```python
from build123d import *

# Parameters (mm, degrees)
SKETCH1_W                       = 950
SKETCH1_H                       = 200
BASE_FLANGE1_DEPTH              = 10
EDGE_FLANGE1_STRIP_W            = 41.4732
EDGE_FLANGE1_STRIP_H            = 10
EDGE_FLANGE1_STRIP_CUT_DEPTH    = 200
EDGE_FLANGE1_STRIP_2_W          = 41.4732
EDGE_FLANGE1_STRIP_2_H          = 10
EDGE_FLANGE1_STRIP_CUT_2_DEPTH  = 200
EDGE_FLANGE1_DEPTH              = 200
EDGE_FLANGE1_BEND_DEPTH         = 200
BREAK_CORNER1_START             = -475
BREAK_CORNER1_DEPTH             = 950
M10_CLEARANCE_HOLE1_D           = 12
M10_CLEARANCE_HOLE1_CSINK_D     = 12.05
M10_CLEARANCE_HOLE1_CSINK_ANGLE = 90
M10_CLEARANCE_HOLE2_D           = 12
M10_CLEARANCE_HOLE2_CSINK_D     = 12.05
M10_CLEARANCE_HOLE2_CSINK_ANGLE = 90
FILLET1_R                       = 3


# Read off the part's stored shape, not the designer's step: Break-Corner1
# Sheet-metal steps are written as plain solids
with BuildPart() as part:
    # Sketch1 → Base-Flange1 (new body)
    with BuildSketch(Plane(origin=(0, 0, 0), x_dir=(1, 0, 0), z_dir=(0, 1, 0))):
        Rectangle(SKETCH1_W, SKETCH1_H)
    extrude(amount=-BASE_FLANGE1_DEPTH)

    # Edge-Flange1 strip (across the edge) → Edge-Flange1 strip cut (cut)
    with BuildSketch(Plane(origin=(-475, 0, -100), x_dir=(1, 0, 0), z_dir=(0, 0, 1))):
        with Locations((-10, -5)):
            Rectangle(EDGE_FLANGE1_STRIP_W, EDGE_FLANGE1_STRIP_H)
    extrude(amount=EDGE_FLANGE1_STRIP_CUT_DEPTH, mode=Mode.SUBTRACT)

    # Edge-Flange1 strip 2 (across the edge) → Edge-Flange1 strip cut 2 (cut)
    with BuildSketch(Plane(origin=(475, 0, 100), x_dir=(-1, 0, 0), z_dir=(0, 0, -1))):
        with Locations((-10, -5)):
            Rectangle(EDGE_FLANGE1_STRIP_2_W, EDGE_FLANGE1_STRIP_2_H)
    extrude(amount=EDGE_FLANGE1_STRIP_CUT_2_DEPTH, mode=Mode.SUBTRACT)

    # Edge-Flange1 section (across the edge) → Edge-Flange1 (add)
    with BuildSketch(Plane(origin=(-475, 0, -100), x_dir=(1, 0, 0), z_dir=(0, 0, 1))):
        with BuildLine():
            Line((0, 0.7366), (0, 115))
            Line((0, 115), (10, 115))
            Line((10, 115), (10, 0.7366))
            ThreePointArc((10, 0.7366), (10.215745145, 0.215745145), (10.7366, 0))
            Line((10.7366, 0), (10.7366, -10))
            ThreePointArc((10.7366, -10), (3.144677333, -6.855322667), (0, 0.7366))
        make_face()
    extrude(amount=EDGE_FLANGE1_DEPTH)

    # Edge-Flange1 section 2 (across the edge) → Edge-Flange1 bend (add)
    with BuildSketch(Plane(origin=(475, 0, 100), x_dir=(-1, 0, 0), z_dir=(0, 0, -1))):
        with BuildLine():
            Line((0, 0.7366), (0, 115))
            Line((0, 115), (10, 115))
            Line((10, 115), (10, 0.7366))
            ThreePointArc((10, 0.7366), (10.215745145, 0.215745145), (10.7366, 0))
            Line((10.7366, 0), (10.7366, -10))
            ThreePointArc((10.7366, -10), (3.144677333, -6.855322667), (0, 0.7366))
        make_face()
    extrude(amount=EDGE_FLANGE1_BEND_DEPTH)

    # Break-Corner1 outline → Break-Corner1 (cut)
    with BuildSketch(Plane.YZ.offset(BREAK_CORNER1_START)):
        Polygon((115, 100), (105, 100), (115, 90), align=None)
        Polygon((115, -100), (115, -90), (105, -100), align=None)
    extrude(amount=BREAK_CORNER1_DEPTH, mode=Mode.SUBTRACT)

    # M10 Clearance Hole1 (through all)
    with Locations(Plane(origin=(475, 60, -70), x_dir=(0, 1, 0), z_dir=(1, 0, 0))):
        with Locations((0, 0), (0, 35), (0, 70), (0, 105), (0, 140), (30, 17.5), (30, 52.5), (30, 87.5), (30, 122.5)):
            CounterSinkHole(M10_CLEARANCE_HOLE1_D / 2, M10_CLEARANCE_HOLE1_CSINK_D / 2, counter_sink_angle=M10_CLEARANCE_HOLE1_CSINK_ANGLE)

    # M10 Clearance Hole2 (through all)
    with Locations(Plane(origin=(0, 0, 0), x_dir=(1, 0, 0), z_dir=(0, 1, 0))):
        with Locations((330, 40), (270, 40), (210, 40), (150, 40), (330, 0), (330, -40), (270, -40), (210, -40), (150, -40)):
            m10_clearance_hole2 = CounterSinkHole(M10_CLEARANCE_HOLE2_D / 2, M10_CLEARANCE_HOLE2_CSINK_D / 2, counter_sink_angle=M10_CLEARANCE_HOLE2_CSINK_ANGLE)

    # Mirror1: M10 Clearance Hole2 across plane
    add(m10_clearance_hole2.mirror(Plane(origin=(0, 0, 0), x_dir=(0, 0, 1), z_dir=(1, 0, 0))), mode=Mode.SUBTRACT)

    # Fillet1
    fillet1_edges = [part.edges().sort_by_distance(p)[0] for p in [
        (465, 110, 95),
        (470, 115, 90),
        (475, 110, 95),
        (0, 0, 100),
        (0, -10, 100),
        (0, 0, -100),
        (0, -10, -100),
        (-471.855322667, -6.855322667, -100),
        (-471.855322667, -6.855322667, 100),
        (-464.784254855, 0.215745145, -100),
        (-464.784254855, 0.215745145, 100),
        (-465, 52.8683, 100),
        (-475, 52.8683, 100),
        (471.855322667, -6.855322667, 100),
        (471.855322667, -6.855322667, -100),
        (464.784254855, 0.215745145, 100),
        (464.784254855, 0.215745145, -100),
        (465, 52.8683, -100),
        (475, 52.8683, -100),
        (-465, 115, 0),
        (-475, 115, 0),
        (-470, 115, 90),
        (-465, 110, 95),
        (-470, 105, 100),
        (-475, 110, 95),
        (-475, 52.8683, -100),
        (-465, 52.8683, -100),
        (-470, 105, -100),
        (-465, 110, -95),
        (-470, 115, -90),
        (-475, 110, -95),
        (465, 115, 0),
        (475, 115, 0),
        (470, 115, -90),
        (465, 110, -95),
        (470, 105, -100),
        (475, 110, -95),
        (475, 52.8683, 100),
        (465, 52.8683, 100),
        (470, 105, 100),
    ]]
    fillet(fillet1_edges, radius=FILLET1_R)


solid = part.part
```
Here's how the part is built. I have some questions about the finished solid (model axes, mm). A direction names the side the tool comes from. Give positions to 0.01 mm unless a question says otherwise; leave off trailing zeros. Loops run counter-clockwise (first coordinate to the right, second up) from the corner with the lowest first, then second, coordinate; pieces in that order, holes last. Notation, with made-up numbers: (73.25, 86.5) -> (110.25, 86.5) arc R22 ccw to (110.25, 98.5) -> close; hole circle Ø1 at (13, -14). An arc over 180 degrees is marked (long way). Use one line per item in the form item = value. Start each with the question number.
1) Which directions (+Z, -Z, +X, -X, +Y, -Y) give clear straight access to the entire face, cutting with the end or side of a thin tool? Please do faces 4 (the face through (-6, -10, -1)), 5 (the face through (465, 45, 1)).
2) Please list where these lines run through material, in increasing order: line 1 along Z through (x, y) = (472.25, 90); line 2 along Z through (x, y) = (-270, -7); line 3 along Z through (x, y) = (330, -4).
3) Imagine slicing it at A-A (x = 111.5). Please give me the cut outline in (y, z), then the cut area to 3 significant figures.
4) Thinking about a two-plate mould opening in X: for faces 1 (the face through (-2, -5, -100)), 2 (the face through (475, 43, 1)), 3 (the face through (-6, 0, -1)), which applies, +X half, -X half, draft (parallel to the pull), parting line (faces both ways), or undercut?
5) For P1, Ø14, axis at x = -330, z = 0, coming from the -Y side; P2, Ø1.5, axis at x = -155.5, z = 40.5, coming from the +Y side, each with a flat end and sliding along its axis, tell me the tip position at first contact or that it passes through.
Check values:
q1.face_4 = +Z, -Z, +X, -X, -Y
q1.face_5 = +Z, -Z, +Y
q2.line_1 = -99.99 to -58.5, -46.5 to -23.5, -11.5 to 11.5, 23.5 to 46.5, 58.5 to 99.99
q2.line_2 = -100 to -46, -34 to 34, 46 to 100
q2.line_3 = -100 to -46, -34 to -6, 6 to 34, 46 to 100
q3.outline = (-10, -97) arc R3 ccw to (-7, -100) -> (-3, -100) arc R3 ccw to (0, -97) -> (0, 97) arc R3 ccw to (-3, 100) -> (-7, 100) arc R3 ccw to (-10, 97) -> close
q3.area = 1,990 mm^2
q4.face_1 = draft
q4.face_2 = +X half
q4.face_3 = undercut
q5.P1 = -10
q5.P2 = 0
